from build123d import *

# Parameters (mm, degrees)
EXTRUDE_1_DEPTH     = 10
SKETCH_2_R          = 2.5
CUT_EXTRUDE_1_DEPTH = 13.5
HOLE_WIZARD_M4_1_D  = 3.3
CHAMFER_1_SIZE      = 1
CHAMFER_2_SIZE      = 2


with BuildPart() as part:
    # 草图1 → 凸台-拉伸1 (new body)
    with BuildSketch(Plane.XY):
        Polygon((6.75, 0), (6.75, 27), (-6.75, 27), (-6.75, 0), (-2.55, 0), (-2.55, 20), (2.55, 20), (2.55, 0), align=None)
    extrude(amount=EXTRUDE_1_DEPTH)

    # 草图2 → 切除-拉伸1 (cut)
    with BuildSketch(Plane.ZY.offset(6.75)):
        with Locations((5, 6)):
            Circle(SKETCH_2_R)
    extrude(amount=-CUT_EXTRUDE_1_DEPTH, mode=Mode.SUBTRACT)

    # M4 螺纹孔1 (through all)
    with Locations(Plane(origin=(0, 27, 0), x_dir=(1, 0, 0), z_dir=(0, 1, 0))):
        with Locations((0, -5)):
            Hole(HOLE_WIZARD_M4_1_D / 2)

    # 倒角1
    chamfer_1_edges = [part.edges().sort_by_distance(p)[0] for p in [
        (6.75, 0, 5),
        (2.55, 0, 5),
        (-2.55, 0, 5),
        (-6.75, 0, 5),
    ]]
    chamfer(chamfer_1_edges, length=CHAMFER_1_SIZE)

    # 倒角2
    chamfer_2_edges = [part.edges().sort_by_distance(p)[0] for p in [
        (-6.75, 27, 5),
        (6.75, 27, 5),
    ]]
    chamfer(chamfer_2_edges, length=CHAMFER_2_SIZE)


solid = part.part
Geometry: final body of the model. Coordinates: model frame, mm. A direction names the side the tool comes from. Give positions to 0.01 mm unless a question says otherwise; leave off trailing zeros. Order: outer loops, then holes, each group sorted by start corner. A loop starts at its lowest first (then second) coordinate and runs counter-clockwise, first axis right, second up. Notation, with made-up numbers: (-31.5, 44.5) -> (-16.5, 44.5) arc R29 ccw to (-16.5, 80.5) -> close; hole circle Ø1 at (44.25, -20). An arc over 180 degrees is marked (long way). Put each result on its own line as item: value.
Q1. Pin query (flat end, axial travel): pin 1 (3 mm diameter, centred on y = 6, z = 5, fed in from +X); pin 2 (2.5 mm diameter, centred on x = 1, z = 3, fed in from -Y). Return the tip coordinate at first contact, or that it passes through.
Here are the results:
pin 1: passes through
pin 2: stops at y = 20
Q2. Section B-B, the plane x = 0. Return loops of the section in (y, z).
Here are the results:
outline: (20, 0) -> (27, 0) -> (27, 3.35) -> (20, 3.35) -> close; (20, 6.65) -> (27, 6.65) -> (27, 10) -> (20, 10) -> close
Q3. Section A-A, the plane y = 9.75. Return loops of the section in (x, z), then the cut area to 3 significant figures.
Here are the results:
outline: (-6.75, 0) -> (-2.55, 0) -> (-2.55, 10) -> (-6.75, 10) -> close; (2.55, 0) -> (6.75, 0) -> (6.75, 10) -> (2.55, 10) -> close
area: 84.0 mm^2
Q4. Section C-C, the plane y = 6. Return loops of the section in (x, z), then the cut area to 3 significant figures.
Here are the results:
outline: (-6.75, 0) -> (-2.55, 0) -> (-2.55, 2.5) -> (-6.75, 2.5) -> close; (-6.75, 7.5) -> (-2.55, 7.5) -> (-2.55, 10) -> (-6.75, 10) -> close; (2.55, 0) -> (6.75, 0) -> (6.75, 2.5) -> (2.55, 2.5) -> close; (2.55, 7.5) -> (6.75, 7.5) -> (6.75, 10) -> (2.55, 10) -> close
area: 42.0 mm^2
Q5. Reachability of faces 1 (the face through (-2.55, 10, 5)), 2 (the face through (5.74, 26.01, 4.93)) from +Z, -Z, +X, -X, +Y, -Y: full face, straight path, thin tool, end or side. Return the list, or none.
Here are the results:
face 1: +Z, -Z, -Y
face 2: +Z, -Z, +X, +Y
Q6. Section D-D, the plane z = 0.5. Return loops of the section in (x, y).
Here are the results:
outline: (-6.75, 1) -> (-5.75, 0) -> (-3.55, 0) -> (-2.55, 1) -> (-2.55, 20) -> (2.55, 20) -> (2.55, 1) -> (3.55, 0) -> (5.75, 0) -> (6.75, 1) -> (6.75, 25) -> (4.75, 27) -> (-4.75, 27) -> (-6.75, 25) -> close
Q7. Material intervals for L1, parallel to Y at x = -4.4, z = 5; L2, parallel to X at y = 8.75, z = 9.25; L3, parallel to Z at x = 0, y = 22.25, sorted ascending.
Here are the results:
L1: y = 0 to 3.5, 8.5 to 27
L2: x = -6.75 to -2.55, 2.55 to 6.75
L3: z = 0 to 3.35, 6.65 to 10
Q8. Draft query along Z for faces 3 (the face through (0.4, 23.5, 6.6)), 4 (the face through (3, 14, 0)), 5 (the face through (3, 14, 10)), 6 (the face through (-2, 20, 5)). Return one class per face: released by +Z, released by -Z, zero draft, split by the parting line, or undercut.
Here are the results:
face 3: undercut
face 4: released by -Z
face 5: released by +Z
face 6: zero draft
